Answer from the drawing. Dimensions are ordinates in mm from the lowest x, y and z of the part. A direction names the side the tool comes from. Coordinates: 2 decimals unless noted, no trailing zeros. Write each loop counter-clockwise with the first axis right and the second up, starting at its lowest first coordinate (ties: lowest second). Pieces come first, ordered by that corner, then holes. Notation, with made-up numbers: (78, -25.75) -> (103, -25.75) arc R33 cw to (103, 13.25) -> close; hole circle Ø5 at (-25.75, -39.5). An arc over 180 degrees is marked (long way). One line per item, written item: value. Start each with the question number.
1. For a pull along Y with two mould halves and no side action, classify the marked faces 3, 4 and 5 as pulls with the +Y half, pulls with the -Y half, needs draft (parallel to the pull), parting line crosses it, or undercut.
2. For the marked faces 1 and 2, determine the directions among +Z, -Z, +X, -X, +Y, -Y from which every point of the face is accessible in a straight line to the end or side of a thin tool.
3. Consider line 1 along Z through (x, y) = (3, 19.05); line 2 along Z through (x, y) = (10.5, 8.5); line 3 along Z through (x, y) = (2.5, 20). Determine where each line is inside the solid, lowest interval first.
4. Find section B-B, the plane x = 8.5. Write down the section's boundary in (y, z).
5. Given P1, Ø4, axis at x = 5, y = 13, coming from the +Z side; P2, Ø4, axis at x = 4, y = 6.5, coming from the +Z side; P3, Ø5, axis at x = 5, z = 25.5, coming from the -Y side, each flat-ended and moving along its own axis, determine where each tip first touches the part or whether it passes through.
6. Find section D-D, the plane z = 9. Write down the section's boundary in (x, y) (1 decimal).
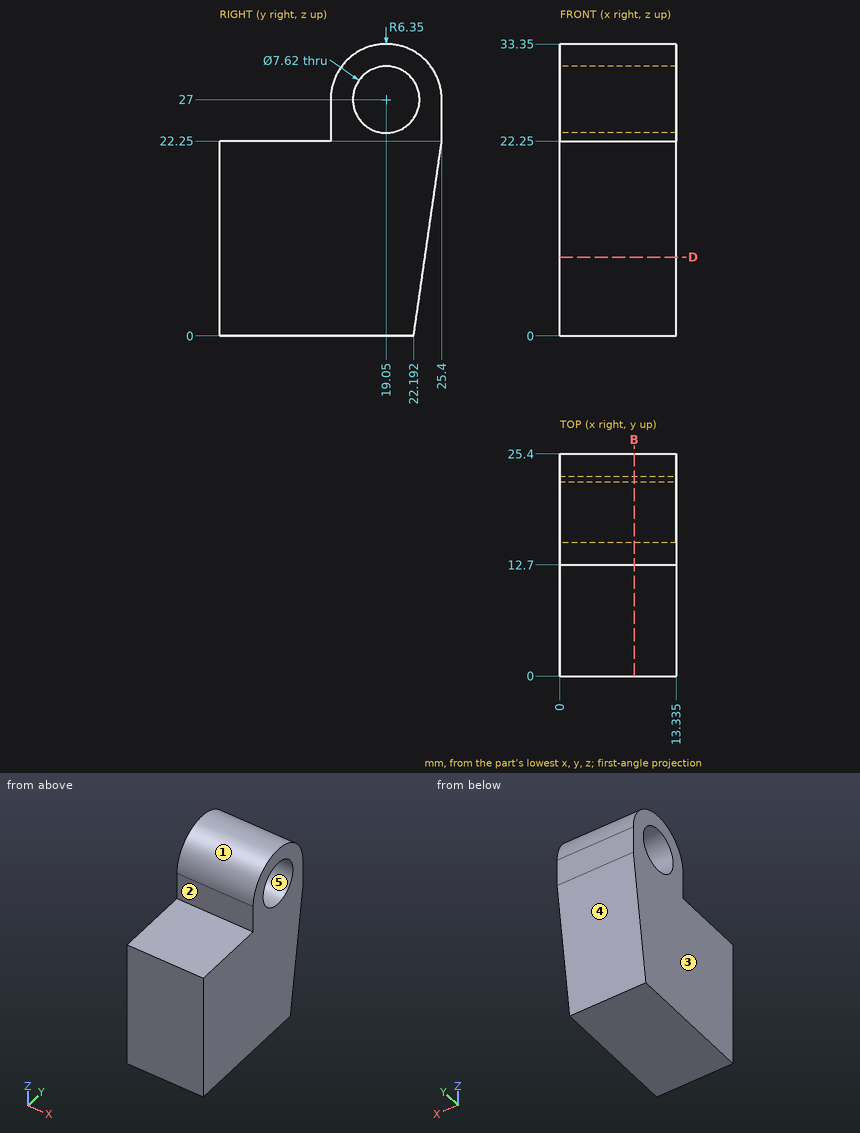
Answer block:
1. face 3: needs draft
1. face 4: pulls with the +Y half
1. face 5: undercut
2. face 1: +Z, +X, -X
2. face 2: +Z, +X, -X, -Y
3. line 1: z = 0 to 23.19, 30.81 to 33.35
3. line 2: z = 0 to 22.25
3. line 3: z = 0 to 23.31, 30.69 to 33.28
4. outline: (0, 0) -> (22.19, 0) -> (25.4, 22.25) -> (25.4, 27) arc R6.35 ccw to (12.7, 27) -> (12.7, 22.25) -> (0, 22.25) -> close; hole circle Ø7.62 at (19.05, 27)
5. P1: stops at z = 31.89
5. P2: stops at z = 22.25
5. P3: stops at y = 12.7
6. outline: (0, 0) -> (13.3, 0) -> (13.3, 23.5) -> (0, 23.5) -> close
